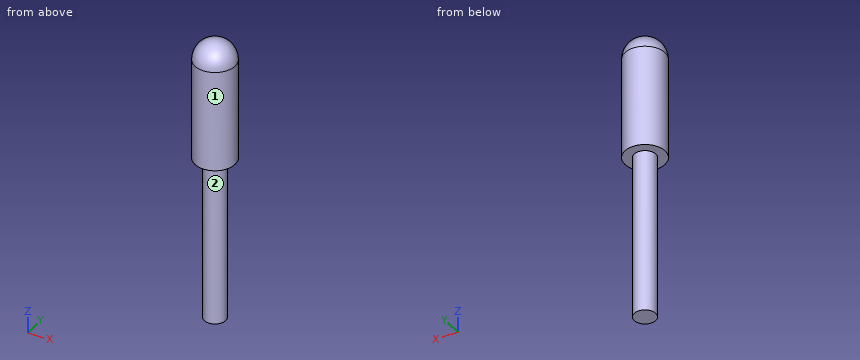
Autodesk Inventor part; units mm, degrees
ref_plane "YZ Plane" through (0, 0, 0) normal (1, 0, 0) x (0, 1, 0)
ref_plane "XZ Plane" through (0, 0, 0) normal (0, 1, 0) x (-1, 0, 0)
ref_plane "XY Plane" through (0, 0, 0) normal (0, 0, 1) x (1, 0, 0)
sketch "Sketch1" plane through (0, 0, 0) normal (0, 0, 1) x (1, 0, 0)
  circle A0 centre (0, 0) radius 6
  dimension "d0" = 12
extrude "Extrusion1" add sketch "Sketch1" along normal blind 24.38 and the other way blind 10
fillet "Fillet1" radius 6 1 edges at (-6, 0, 24.38)
sketch "Sketch2" plane through (0, 0, -10) normal (0, 0, -1) x (-1, 0, 0)
  circle A0 centre (0, 0) radius 3.4
  dimension "d6" = 6.8
extrude "Extrusion2" add sketch "Sketch2" along normal blind 46
thicken "Thicken1" operation add thickness 0.4 both sides no extend neighbours yes toward (-0.9870503, 0.1604113, 0) faces at (5.9223, -0.9625, 12.2533) (5.9223, -0.9625, -6.6667) (-5.8689, 0, 19.6275)
thicken "Thicken2" operation add thickness 0.4 both sides no extend neighbours yes toward (0.9967573, -0.0804666, 0) faces at (-3.389, 0.2736, -25.3333)
properties part number "SpringRod"
The model under review builds one solid part; all positions refer to its coordinate system, in mm. Face numbers are marked on the shaded views. A direction names the side the tool comes from. Give positions to 0.01 mm unless a question says otherwise; leave off trailing zeros. Write each loop counter-clockwise with the first axis right and the second up, starting at its lowest first coordinate (ties: lowest second). Pieces come first, ordered by that corner, then holes.
(1) Tool access review of the marked faces 1 and 2: name each direction out of +Z, -Z, +X, -X, +Y, -Y from which nothing blocks a thin tool from reaching the whole face with its end or side.
(2) Consider section C-C, the plane z = -48.5. Give the boundary of the cut face in (x, y), and give its area (3 significant figures).
(3) Consider section A-A, the plane x = 0. Give the boundary of the cut face in (y, z).
(4) Consider section D-D, the plane x = 4.5. Give the boundary of the cut face in (y, z).
(5) For P1, Ø3, axis at y = 3, z = -41.5, coming from the +X side; P2, Ø1.5, axis at x = -3.5, z = -10.5, coming from the +Y side; P3, Ø2, axis at x = -2.5, y = -3, coming from the +Z side, all flat-tipped, find the tip position at first contact; note any pin that passes through.
(6) To check wall thickness, follow L1, parallel to Y at x = 0, z = -12; L2, parallel to Z at x = -3.75, y = -1.5; L3, parallel to Y at x = 2, z = -49. State the ranges of each line that lie inside material, in increasing order.
Returned:
1. face 1: +Z, -Z
1. face 2: -Z
2. outline: circle Ø6 at (0, 0)
2. area: 28.3 mm2
3. outline: (-5.6, -10) - (-3, -10) - (-3, -56) - (3, -56) - (3, -10) - (5.6, -10) - (5.6, 18.38) arc R5.6 ccw to (-5.6, 18.38) - close
4. outline: (-3.33, -10) - (3.33, -10) - (3.33, 18.38) arc R3.33 ccw to (-3.33, 18.38) - close
5. P1: stops at x = 2.6
5. P2: stops at y = 4.77
5. P3: stops at z = 23.17
6. L1: y = -3 to 3
6. L2: z = -10 to 22.26
6. L3: y = -2.24 to 2.24
